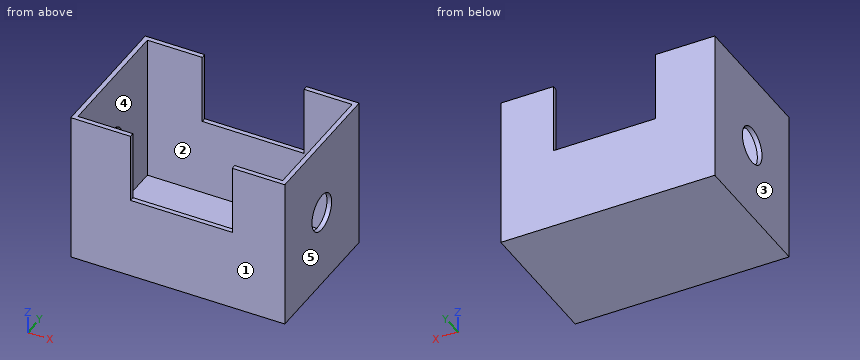
```python
from build123d import *

# Parameters (mm, degrees)
F1_DEPTH = 76.2
F2_T     = -2.54
F3_R     = 10.061541377
F4_DEPTH = 117.1720453928


with BuildPart() as f1:
    # F0 (on Front) → F1 (new body)
    with BuildSketch(Plane.XZ):
        Polygon((-20.8796709776, 51.1912330985), (-53.4663982689, 51.1912330985), (-53.4663982689, -31.8523235619), (63.7046471238, -31.8523235619), (63.7046471238, 51.1912330985), (34.9526293576, 51.1912330985), (34.9526293576, 12.9971429706), (-20.8796709776, 12.9971429706), align=None)
    extrude(amount=F1_DEPTH)

    # F2
    f2_openings = [f1.faces().sort_by_distance(p)[0] for p in [
        (-37.173035, -38.1, 51.191233),
        (49.328638, -38.1, 51.191233),
        (-20.879671, -38.1, 32.094188),
        (7.036479, -38.1, 12.997143),
        (34.952629, -38.1, 32.094188),
    ]]
    offset(amount=F2_T, openings=f2_openings)

    # F3 (on face) → F4 (cut, through all)
    with BuildSketch(Plane.YZ.offset(63.7046471238)):
        with Locations((-38.298625499, 10.4278437793)):
            Circle(F3_R)
    extrude(amount=-F4_DEPTH, mode=Mode.SUBTRACT)


solid = f1.part
```
Verification items for the finished model (mm, model axes). Face numbers are marked on the shaded views. A direction names the side the tool comes from. Give positions to 0.01 mm unless a question says otherwise; leave off trailing zeros. Order: outer loops, then holes, each group sorted by start corner. A loop starts at its lowest first (then second) coordinate and runs counter-clockwise, first axis right, second up. Notation, with made-up numbers: M -16,43.25 L 10,43.25 A25 cw 10,82.25 Z; hole C 85,20 d7. An arc over 180 degrees is marked long. Return JSON: item names as keys, results as strings. Group by question number.
1) Section check A-A on z = 37. Record the cut outline in (x, y), and give its area (3 significant figures).
2) Go/stop test with flat-tipped pins: pin 1 Ø1.3 at (x, y) = (16, -1) entering from +Z; pin 2 Ø6 at (x, z) = (-10.5, -14.5) entering from +Y; pin 3 Ø4 at (x, y) = (-9.5, -22.5) entering from +Z. Record where each tip stops, or that it passes through.
3) Section check B-B on x = -33.5. Record the cut outline in (y, z), and give its area (3 significant figures).
4) Scan lines: line 1 (X direction, y = -71.5, z = 10); line 2 (Y direction, x = -16.5, z = -7); line 3 (Z direction, x = 30, y = -7). Record each from-to range of solid material in increasing order.
5) Section check D-D on z = -7.5. Record the cut outline in (x, y).
6) Mould release check, pull along X, two halves, no side actions. Record for the marked faces 3, 4 and 5: pulls with the +X half, pulls with the -X half, needs draft (parallel to the pull), parting line crosses it, or undercut.
7) Section check C-C on y = -31.5. Record the cut outline in (x, z), and give its area (3 significant figures).
8) Access from +Z, -Z, +X, -X, +Y, -Y to the whole of each face (thin tool, end or side, straight path). Record for the marked faces 1 and 2.
Answer block:
{
 "1": {"outline": "M -53.47,-76.2 L -20.88,-76.2 L -20.88,-73.66 L -50.93,-73.66 L -50.93,-2.54 L -20.88,-2.54 L -20.88,0 L -53.47,0 Z; M 34.95,-76.2 L 63.7,-76.2 L 63.7,0 L 34.95,0 L 34.95,-2.54 L 61.16,-2.54 L 61.16,-73.66 L 34.95,-73.66 Z", "area": "673 mm^2"},
 "2": {"pin 1": "stops at z = 13", "pin 2": "stops at y = 0", "pin 3": "stops at z = -29.31"},
 "3": {"outline": "M -76.2,-31.85 L 0,-31.85 L 0,51.19 L -2.54,51.19 L -2.54,-29.31 L -73.66,-29.31 L -73.66,51.19 L -76.2,51.19 Z", "area": "603 mm^2"},
 "4": {"line 1": "x = -53.47 to -50.93, 61.16 to 63.7", "line 2": "y = -76.2 to -73.66, -2.54 to 0", "line 3": "z = -31.85 to -29.31"},
 "5": {"outline": "M -53.47,-76.2 L 63.7,-76.2 L 63.7,0 L -53.47,0 Z; hole M -50.93,-73.66 L 61.16,-73.66 L 61.16,-2.54 L -50.93,-2.54 Z"},
 "6": {"face 3": "pulls with the -X half", "face 4": "undercut", "face 5": "pulls with the +X half"},
 "7": {"outline": "M -53.47,-31.85 L 63.7,-31.85 L 63.7,3.01 L 61.16,3.01 L 61.16,-29.31 L -50.93,-29.31 L -50.93,3.01 L -53.47,3.01 Z; M -53.47,17.84 L -50.93,17.84 L -50.93,51.19 L -53.47,51.19 Z; M 61.16,17.84 L 63.7,17.84 L 63.7,51.19 L 61.16,51.19 Z", "area": "631 mm^2"},
 "8": {"face 1": "+Z, -Z, +X, -X, -Y", "face 2": "+Z"}
}
